from build123d import *

# Parameters (mm, degrees)
ESQUISSE1_R        = 1.5
BOSS_EXTRU_1_DEPTH = 1.6
ESQUISSE2_W        = 2
ESQUISSE2_H        = 4
BOSS_EXTRU_2_DEPTH = 1


with BuildPart() as part:
    # Esquisse1 → Boss.-Extru.1 (new body)
    with BuildSketch(Plane.XY):
        with BuildLine():
            Line((6.5, -3.5), (6.5, -11.5))
            ThreePointArc((6.5, -11.5), (0, -18), (-6.5, -11.5))
            Line((-6.5, -11.5), (-6.5, -3.5))
            ThreePointArc((-6.5, -3.5), (0, 3), (6.5, -3.5))
        make_face()
        with Locations((0, -15)):
            Circle(ESQUISSE1_R, mode=Mode.SUBTRACT)
    extrude(amount=BOSS_EXTRU_1_DEPTH)

    # Esquisse2 → Boss.-Extru.2 (add)
    with BuildSketch(Plane.XY.offset(1.6)):
        Rectangle(ESQUISSE2_W, ESQUISSE2_H)
    extrude(amount=BOSS_EXTRU_2_DEPTH)


solid = part.part
Read the model definition and answer for the solid it produces. Units are mm, in the model's axes. A direction names the side the tool comes from. Give positions to 0.01 mm unless a question says otherwise; leave off trailing zeros. Write each loop counter-clockwise with the first axis right and the second up, starting at its lowest first coordinate (ties: lowest second). Pieces come first, ordered by that corner, then holes. Notation, with made-up numbers: (38.5, -22.75) - (74.5, -22.75) arc R7 cw to (74.5, -15.75) - close; hole circle Ø3 at (45, 49.5). An arc over 180 degrees is marked (long way). Use CSV: the item, a comma, the result in double quotes. Start each with the question number.
Item 1: For faces 1 (the flat face through (6.5, -7, 1)), 2 (the cylindrical face through (0, 3, 1)), 3 (the flat face through (0, -2, 2)), 4 (the flat face through (-1, 0, 2)), 5 (the flat face through (1, 0, 2)), determine the directions among +Z, -Z, +X, -X, +Y, -Y from which every point of the face is accessible in a straight line to the end or side of a thin tool.
Item 2: The part is cut by section B-B, the plane y = -15. Give the vertices of the cut face in (x, z), and give its area (3 significant figures).
Item 3: The part is cut by section D-D, the plane y = 1. Give the vertices of the cut face in (x, z), and give its area (3 significant figures).
Item 4: The part is cut by section C-C, the plane z = 0.95. Give the vertices of the cut face in (x, y).
Item 5: The mould has two halves that part along Y. Classify faces 6 (the cylindrical face through (-0.325, -16.464, 0.789)), 7 (the flat face through (0, 0, 2.6)), 8 (the flat face through (0, 2, 2)): pulls with the +Y half, pulls with the -Y half, needs draft (parallel to the pull), parting line crosses it, or undercut.
Item 6: The part is cut by section A-A, the plane x = 0. Give the vertices of the cut face in (y, z).
Item 7: Consider line 1 (Y direction, x = 0, z = 0.5); line 2 (Z direction, x = -0.5, y = -9.25); line 3 (Y direction, x = 0.5, z = 2.2). Determine where each line is inside the solid, lowest interval first.
Item 8: Flat-ended cylindrical pins translate along their axes: P1, Ø1.5, axis at x = -3.5, z = 2, coming from the +Y side; P2, Ø1.1, axis at x = 0, z = 2, coming from the +Y side; P3, Ø4, axis at x = 0, y = -15, coming from the +Z side; P4, Ø0.5, axis at x = 0.5, z = 2, coming from the -Y side. Find the tip coordinate at first contact, or state that the pin passes through.
Taken from the geometry:
1,face 1,"+Z, -Z, +X, +Y, -Y"
1,face 2,"+Z, -Z, +Y"
1,face 3,"+Z, +X, -X, -Y"
1,face 4,"+Z, -X, +Y, -Y"
1,face 5,"+Z, +X, +Y, -Y"
2,outline,"(-5.48, 0) - (-1.5, 0) - (-1.5, 1.6) - (-5.48, 1.6) - close; (1.5, 0) - (5.48, 0) - (5.48, 1.6) - (1.5, 1.6) - close"
2,area,"12.7 mm2"
3,outline,"(-4.69, 0) - (4.69, 0) - (4.69, 1.6) - (1, 1.6) - (1, 2.6) - (-1, 2.6) - (-1, 1.6) - (-4.69, 1.6) - close"
3,area,"17.0 mm2"
4,outline,"(-6.5, -11.5) arc R6.5 ccw to (6.5, -11.5) - (6.5, -3.5) arc R6.5 ccw to (-6.5, -3.5) - close; hole circle Ø3 at (0, -15)"
5,face 6,"undercut"
5,face 7,"needs draft"
5,face 8,"pulls with the +Y half"
6,outline,"(-18, 0) - (-16.5, 0) - (-16.5, 1.6) - (-18, 1.6) - close; (-13.5, 0) - (3, 0) - (3, 1.6) - (2, 1.6) - (2, 2.6) - (-2, 2.6) - (-2, 1.6) - (-13.5, 1.6) - close"
7,line 1,"-18 to -16.5, -13.5 to 3"
7,line 2,"0 to 1.6"
7,line 3,"-2 to 2"
8,P1,"y = 2.33"
8,P2,"y = 3"
8,P3,"z = 1.6"
8,P4,"y = -2"
